Could you check a few things on this model? Use its own coordinates, in mm. A direction names the side the tool comes from. Round coordinates to 2 decimals unless told otherwise and drop trailing zeros. Write each loop counter-clockwise with the first axis right and the second up, starting at its lowest first coordinate (ties: lowest second). Pieces come first, ordered by that corner, then holes. Notation, with made-up numbers: (51, -5.75) -> (69, -5.75) arc R18 ccw to (69, 3.25) -> close; hole circle Ø11 at (14, 79). An arc over 180 degrees is marked (long way). Answer in a Markdown table with one row per item.
Autodesk Inventor part; units mm, degrees
ref_plane "Work Plane1" through (0, 0, -55) normal (0, 0, 1) x (1, 0, 0)
ref_plane "YZ Plane" through (0, 0, 0) normal (1, 0, 0) x (0, 1, 0)
ref_plane "XZ Plane" through (0, 0, 0) normal (0, 1, 0) x (-1, 0, 0)
sketch "Sketch1" plane through (0, 0, 0) normal (0, 0, 1) x (1, 0, 0)
  circle A0 centre (0, 0) radius 8
  dimension "d0" = 16
sketch "Sketch2" plane through (0, 0, 0) normal (0, 1, 0) x (-1, 0, 0)
  line L0 (0, 0) -> (0, -22)
  line L1 (-20, -42) -> (-85, -42)
  line L2 (-105, -22) -> (-105, 0)
  arc A0 (-20, -42) -> (0, -22) centre (-20, -22) ccw
  arc A1 (-105, -22) -> (-85, -42) centre (-85, -22) ccw
  point P0 (0, -42)
  point P1 (-105, -42)
  dimension "d1" = 105
  dimension "d2" = 42
  dimension "d3" = 20
sweep "Sweep1" add profiles "Sketch1" path "Sketch2"
ref_plane "Work Plane1" through (0, 0, -55) normal (0, 0, 1) x (1, 0, 0)
sketch "Sketch3" plane through (0, 0, -55) normal (0, 0, 1) x (1, 0, 0)
  circle A0 centre (0, 0) radius 3.7
  circle A1 centre (105, 0) radius 8
  circle A2 centre (105, 0) radius 3.7
  dimension "d7" = 7.4
  dimension "d8" = 7.4
extrude "Extrusion1" cut sketch "Sketch3" along normal blind 49 contours A0 | A2
sketch "Sketch4" plane through (0, 0, -6) normal (0, 0, -1) x (-1, 0, 0)
  circle A0 centre (0, 0) radius 3.7
  circle A1 centre (-105, 0) radius 3.7
  circle A2 centre (0, 0) radius 2.25
  circle A3 centre (-105, 0) radius 2.25
  dimension "d11" = 4.5
  dimension "d12" = 4.5
extrude "Extrusion2" cut sketch "Sketch4" against normal up to surface (6 mm away) contours A2 | A3
properties part number "FrameHandle" material "ABS Plastic"
1) Imagine slicing it at B-B, the plane y = 5.75. Please give me the cut outline in (x, z), plus the area to 3 significant figures.
Findings:
| item | result |
|---|---|
| outline | (-5.56, -22) arc R25.56 ccw to (20, -47.56) -> (85, -47.56) arc R25.56 ccw to (110.56, -22) -> (110.56, 0) -> (99.44, 0) -> (99.44, -22) arc R14.44 cw to (85, -36.44) -> (20, -36.44) arc R14.44 cw to (5.56, -22) -> (5.56, 0) -> (-5.56, 0) -> close |
| area | 1,910 mm^2 |
2) Please list where these lines run through material, in increasing order: line 1 (Y direction, x = 0, z = -4.1); line 2 (X direction, y = 0, z = -29); line 3 (X direction, y = 2.5, z = -9).
Findings:
| item | result |
|---|---|
| line 1 | y = -8 to -2.25, 2.25 to 8 |
| line 2 | x = -7.11 to -3.7, 3.7 to 10.25, 94.75 to 101.3, 108.7 to 112.11 |
| line 3 | x = -7.6 to -2.73, 2.73 to 7.6, 97.4 to 102.27, 107.73 to 112.6 |
3) For faces 1 (the face through (-1.73, 7.81, -11.15)), 2 (the face through (52.955, 4.868, -48.349)), 3 (the face through (3.418, 1.417, -21.347)), 4 (the face through (0.29, 2.23, -3.04)), which set-ups out of +Z, -Z, +X, -X, +Y, -Y let a thin tool reach every point of the face, with its end or its side?
Findings:
| item | result |
|---|---|
| face 1 | +Z |
| face 2 | none |
| face 3 | -Z |
| face 4 | +Z, -Z |
4) Thinking about a two-plate mould opening in X: for faces 5 (the face through (102.92, -0.86, -3.04)), 6 (the face through (103, -2, 0)), which applies, +X half, -X half, draft (parallel to the pull), parting line (faces both ways), or undercut?
Findings:
| item | result |
|---|---|
| face 5 | undercut |
| face 6 | draft |
5) Imagine slicing it at A-A, the plane y = 0. Please give me the cut outline in (x, z), plus the area to 3 significant figures.
Findings:
| item | result |
|---|---|
| outline | (-8, -22) arc R28 ccw to (-3.7, -36.91) -> (-3.7, -6) -> (-2.25, -6) -> (-2.25, 0) -> (-8, 0) -> close; (2.25, -6) -> (3.7, -6) -> (3.7, -44.77) arc R28 ccw to (20, -50) -> (85, -50) arc R28 ccw to (101.3, -44.77) -> (101.3, -6) -> (102.75, -6) -> (102.75, 0) -> (97, 0) -> (97, -22) arc R12 cw to (85, -34) -> (20, -34) arc R12 cw to (8, -22) -> (8, 0) -> (2.25, 0) -> close; (107.25, -6) -> (108.7, -6) -> (108.7, -36.91) arc R28 ccw to (113, -22) -> (113, 0) -> (107.25, 0) -> close |
| area | 2,170 mm^2 |
6) Imagine slicing it at C-C, the plane x = 51. Please give me the cut outline in (y, z), plus the area to 3 significant figures.
Findings:
| item | result |
|---|---|
| outline | circle Ø16 at (0, -42) |
| area | 201 mm^2 |
7) For pin 1 (2 mm diameter, centred on x = 104, y = -0.5, fed in from -Z); pin 2 (8 mm diameter, centred on y = 4, z = -23.5, fed in from -X); pin 3 (3 mm diameter, centred on y = -5.5, z = -42, fed in from +X); pin 4 (8 mm diameter, centred on y = 6, z = -14.5, fed in from -X), each with a flat end and sliding along its axis, tell me the tip position at first contact or that it passes through.
Findings:
| item | result |
|---|---|
| pin 1 | passes through |
| pin 2 | stops at x = -8 |
| pin 3 | stops at x = 103.76 |
| pin 4 | stops at x = -7.75 |
